from build123d import *

# Parameters (mm, degrees)
CROQUIS2_W               = 40
CROQUIS2_H               = 55
CROQUIS2_R               = 2
SALIENTE_EXTRUIR1_DEPTH  = 2
CROQUIS3_W               = 40
CROQUIS3_H               = 2
SALIENTE_EXTRUIR2_DEPTH  = 42
CROQUIS4_R               = 3
SALIENTE_EXTRUIR3_DEPTH  = 2
MATRIZL1_COUNT           = 2
MATRIZL1_PITCH           = 12
CROQUIS6_W               = 40
CROQUIS6_H               = 27.5
CORTAR_EXTRUIR1_DEPTH    = 79.89866919
CROQUIS7_W               = 40
CROQUIS7_H               = 2
SALIENTE_EXTRUIR5_DEPTH  = 20
MATRIZL2_COPY_1_SKETCH_R = 3
MATRIZL2_COPY_1_DEPTH    = 2
MATRIZL2_COPY_2_SKETCH_R = 3
MATRIZL2_COPY_2_DEPTH    = 2


with BuildPart() as part:
    # Croquis2 → Saliente-Extruir1 (new body)
    with BuildSketch(Plane(origin=(0, 0, 0), x_dir=(1, 0, 0), z_dir=(0, 1, 0))):
        with Locations((20, 27.5)):
            Rectangle(CROQUIS2_W, CROQUIS2_H)
        with Locations(Location((5, 47.5, 0), (0, 0, 270))):
            Circle(CROQUIS2_R, mode=Mode.SUBTRACT)
        with Locations(Location((35, 47.5, 0), (0, 0, 270))):
            Circle(CROQUIS2_R, mode=Mode.SUBTRACT)
        with Locations(Location((35, 7.5, 0), (0, 0, 270))):
            Circle(CROQUIS2_R, mode=Mode.SUBTRACT)
        with Locations(Location((5, 7.5, 0), (0, 0, 270))):
            Circle(CROQUIS2_R, mode=Mode.SUBTRACT)
    extrude(amount=SALIENTE_EXTRUIR1_DEPTH)

    # Croquis3 → Saliente-Extruir2 (add)
    with BuildSketch(Plane(origin=(0, 0, 0), x_dir=(1, 0, 0), z_dir=(0, 1, 0))):
        with Locations((20, -1)):
            Rectangle(CROQUIS3_W, CROQUIS3_H)
    extrude(amount=SALIENTE_EXTRUIR2_DEPTH)

    # Croquis4 → Saliente-Extruir3 (add)
    with BuildSketch(Plane(origin=(0, 22, 0), x_dir=(1, 0, 0), z_dir=(0, 1, 0))):
        with BuildLine():
            Line((40, 7), (40, 0))
            Line((40, 0), (28, 0))
            Line((28, 0), (28, 7))
            ThreePointArc((28, 7), (34, 13), (40, 7))
        make_face()
        with Locations(Location((34, 7, 0), (0, 0, 270))):
            Circle(CROQUIS4_R, mode=Mode.SUBTRACT)
    saliente_extruir3 = extrude(amount=SALIENTE_EXTRUIR3_DEPTH)

    # MatrizL1: Saliente-Extruir3 ×2
    with Locations(*[(0, -i * MATRIZL1_PITCH, 0) for i in range(1, MATRIZL1_COUNT)]):
        add(saliente_extruir3)

    # Croquis6 → Cortar-Extruir1 (cut, through all)
    with BuildSketch(Plane(origin=(0, 2, 0), x_dir=(1, 0, 0), z_dir=(0, 1, 0))):
        with Locations((20, 41.25)):
            Rectangle(CROQUIS6_W, CROQUIS6_H)
    extrude(amount=-CORTAR_EXTRUIR1_DEPTH, mode=Mode.SUBTRACT)

    # Croquis7 → Saliente-Extruir5 (add)
    with BuildSketch(Plane(origin=(0, 42, 0), x_dir=(1, 0, 0), z_dir=(0, 1, 0))):
        with Locations((20, -1)):
            Rectangle(CROQUIS7_W, CROQUIS7_H)
    extrude(amount=SALIENTE_EXTRUIR5_DEPTH)

    # MatrizL2 copy 1 sketch → MatrizL2 copy 1 (add)
    with BuildSketch(Plane(origin=(0, 41, 0), x_dir=(1, 0, 0), z_dir=(0, 1, 0))):
        with BuildLine():
            Line((40, 7), (40, 0))
            Line((40, 0), (28, 0))
            Line((28, 0), (28, 7))
            ThreePointArc((28, 7), (34, 13), (40, 7))
        make_face()
        with Locations(Location((34, 7, 0), (0, 0, 270))):
            Circle(MATRIZL2_COPY_1_SKETCH_R, mode=Mode.SUBTRACT)
    extrude(amount=MATRIZL2_COPY_1_DEPTH)

    # MatrizL2 copy 2 sketch → MatrizL2 copy 2 (add)
    with BuildSketch(Plane(origin=(0, 53, 0), x_dir=(1, 0, 0), z_dir=(0, 1, 0))):
        with BuildLine():
            Line((40, 7), (40, 0))
            Line((40, 0), (28, 0))
            Line((28, 0), (28, 7))
            ThreePointArc((28, 7), (34, 13), (40, 7))
        make_face()
        with Locations(Location((34, 7, 0), (0, 0, 270))):
            Circle(MATRIZL2_COPY_2_SKETCH_R, mode=Mode.SUBTRACT)
    extrude(amount=MATRIZL2_COPY_2_DEPTH)


solid = part.part
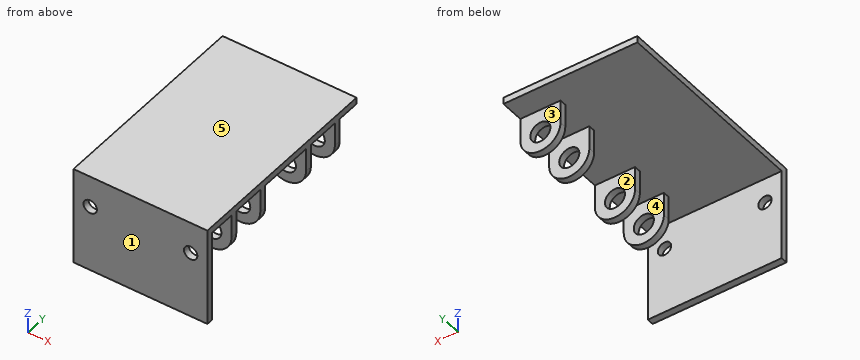
Source: CAD feature listing. Evaluate the final solid. Frame: model axes, mm. Face numbers are marked on the shaded views. A direction names the side the tool comes from. Round coordinates to 2 decimals unless told otherwise and drop trailing zeros. Loops run counter-clockwise (first coordinate to the right, second up) from the corner with the lowest first, then second, coordinate; pieces in that order, holes last. Notation, with made-up numbers: M 27.5,47 L 78.5,47 A15 ccw 78.5,71 Z; hole C 71,-3 d8. An arc over 180 degrees is marked long. Answer as CSV lines item,"result".
Q1. Line query: line 1 along Y through (x, z) = (32.5, -1); line 2 along X through (y, z) = (53.45, -7); line 3 along Z through (x, y) = (38, 58). Output: solid intervals per line, ascending.
Verdict:
line 1,"y = 0 to 2, 10 to 12, 22 to 24, 41 to 43, 53 to 55"
line 2,"x = 28 to 31, 37 to 40"
line 3,"z = 0 to 2"
Q2. Reachability of the marked faces 4 and 5 from +Z, -Z, +X, -X, +Y, -Y: full face, straight path, thin tool, end or side. Return the list, or none.
Verdict:
face 4,"-Z, +X, -X"
face 5,"+Z, +X, -X, +Y, -Y"
Q3. Cut plane B-B (x = 10). Return the cut outline in (y, z).
Verdict:
outline,"M 0,-27.5 L 2,-27.5 L 2,0 L 62,0 L 62,2 L 0,2 Z"
Q4. Cut plane A-A (z = -2.5). Return the cut outline in (x, y).
Verdict:
outline,"M 0,0 L 40,0 L 40,2 L 0,2 Z; M 28,10 L 40,10 L 40,12 L 28,12 Z; M 28,22 L 40,22 L 40,24 L 28,24 Z; M 28,41 L 40,41 L 40,43 L 28,43 Z; M 28,53 L 40,53 L 40,55 L 28,55 Z"
Q5. Contact query for flat-ended pins moving along their axis: pin 1 (5 mm diameter, centred on x = 23.5, y = 24, fed in from -Z); pin 2 (6 mm diameter, centred on x = 31.5, z = -4.5, fed in from +Y); pin 3 (1 mm diameter, centred on y = 54, z = -4, fed in from -X). Output: stop coordinate, or through.
Verdict:
pin 1,"stops at z = 0"
pin 2,"stops at y = 55"
pin 3,"stops at x = 28"
Q6. Pull-direction query (Y, two-part tool) for the marked faces 1, 2 and 3; classes: +Y half, -Y half, draft (parallel to the pull), parting line (faces both ways), or undercut.
Verdict:
face 1,"-Y half"
face 2,"undercut"
face 3,"+Y half"
Q7. Cut plane C-C (y = 7.5). Return the cut outline in (x, z), plus the area to 3 significant figures.
Verdict:
outline,"M 0,0 L 40,0 L 40,2 L 0,2 Z"
area,"80.0 mm^2"
